Verification items for the finished model (mm, model axes). Round coordinates to 2 decimals unless told otherwise and drop trailing zeros. Write each loop counter-clockwise with the first axis right and the second up, starting at its lowest first coordinate (ties: lowest second). Pieces come first, ordered by that corner, then holes. Notation, with made-up numbers: M 28.5,-30.75 L 62.5,-30.75 A19 cw 62.5,-8.75 Z; hole C 33,14.5 d7. An arc over 180 degrees is marked long. Answer in a Markdown table with one row per item. Add a question column.
1. Sectioned sample at B-B on y = -46.99. Record the cut outline in (x, z), plus the area to 3 significant figures.
2. Sectioned sample at C-C on x = 66.04. Record the cut outline in (y, z).
3. Material ranges on probe 1 along Y at (x, z) = (-66.04, 4.25); probe 2 along X at (y, z) = (46.5, 6), recorded low to high.
4. Go/stop test with flat-tipped pins: pin 1 Ø4.5 at (x, y) = (48.36, 8.51) entering from -Z; pin 2 Ø5.5 at (x, y) = (-40.64, -46.99) entering from -Z. Record where each tip stops, or that it passes through.
5. Sectioned sample at A-A on x = -40.64. Record the cut outline in (y, z), plus the area to 3 significant figures.
```python
from build123d import *

# Parameters (mm, degrees)
F0_W     = 152.4
F0_H     = 114.3
F0_R     = 1.6383
F0_R_2   = 1.75
F1_DEPTH = 7.5438
F2_SIZE  = 1.27


with BuildPart() as f1:
    # F0 (on Top) → F1 (new body)
    with BuildSketch(Plane.XY):
        Rectangle(F0_W, F0_H)
        with Locations((-66.04, -46.99)):
            Circle(F0_R, mode=Mode.SUBTRACT)
        with Locations((-40.64, -46.99)):
            Circle(F0_R_2, mode=Mode.SUBTRACT)
        with Locations((66.04, -46.99)):
            Circle(F0_R, mode=Mode.SUBTRACT)
        with Locations((-66.04, 46.99)):
            Circle(F0_R, mode=Mode.SUBTRACT)
        with Locations((48.36, 8.51)):
            Circle(F0_R_2, mode=Mode.SUBTRACT)
        with Locations((66.04, 46.99)):
            Circle(F0_R, mode=Mode.SUBTRACT)
    extrude(amount=F1_DEPTH)

    # F2
    f2_edges = [f1.edges().sort_by_distance(p)[0] for p in [
        (-67.6783, -46.99, 0),
        (-42.39, -46.99, 0),
        (46.61, 8.51, 0),
        (64.4017, 46.99, 0),
        (64.4017, -46.99, 0),
        (-67.6783, 46.99, 0),
    ]]
    chamfer(f2_edges, length=F2_SIZE)


solid = f1.part
```
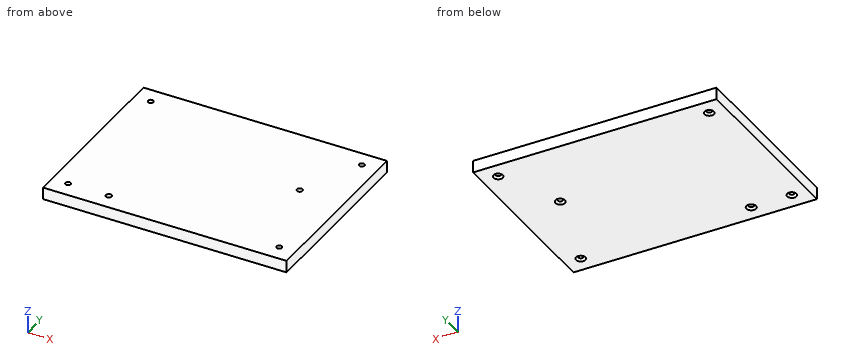
Geometry check:
| question | item | result |
|---|---|---|
| 1 | outline | M -76.2,0 L -68.95,0 L -67.68,1.27 L -67.68,7.54 L -76.2,7.54 Z; M -64.4,1.27 L -63.13,0 L -43.66,0 L -42.39,1.27 L -42.39,7.54 L -64.4,7.54 Z; M -38.89,1.27 L -37.62,0 L 63.13,0 L 64.4,1.27 L 64.4,7.54 L -38.89,7.54 Z; M 67.68,1.27 L 68.95,0 L 76.2,0 L 76.2,7.54 L 67.68,7.54 Z |
| 1 | area | 1,070 mm2 |
| 2 | outline | M -57.15,0 L -49.9,0 L -48.63,1.27 L -48.63,7.54 L -57.15,7.54 Z; M -45.35,1.27 L -44.08,0 L 44.08,0 L 45.35,1.27 L 45.35,7.54 L -45.35,7.54 Z; M 48.63,1.27 L 49.9,0 L 57.15,0 L 57.15,7.54 L 48.63,7.54 Z |
| 3 | probe 1 | y = -57.15 to -48.63, -45.35 to 45.35, 48.63 to 57.15 |
| 3 | probe 2 | x = -76.2 to -67.6, -64.48 to 64.48, 67.6 to 76.2 |
| 4 | pin 1 | stops at z = 0.77 |
| 4 | pin 2 | stops at z = 0.27 |
| 5 | outline | M -57.15,0 L -50.01,0 L -48.74,1.27 L -48.74,7.54 L -57.15,7.54 Z; M -45.24,1.27 L -43.97,0 L 57.15,0 L 57.15,7.54 L -45.24,7.54 Z |
| 5 | area | 834 mm2 |
